For this review, take the finished solid that the model builds, in its own axes (mm). A direction names the side the tool comes from. Give positions to 0.01 mm unless a question says otherwise; leave off trailing zeros. Order: outer loops, then holes, each group sorted by start corner. A loop starts at its lowest first (then second) coordinate and runs counter-clockwise, first axis right, second up. Notation, with made-up numbers: (-8.75, 62.5) - (33.25, 62.5) arc R10 ccw to (33.25, 80.5) - close; hole circle Ø7 at (-31.5, -6). An arc over 180 degrees is marked (long way). One line per item, written item: value.
```python
from build123d import *

# Parameters (mm, degrees)
F0_R         = 25
F1_DEPTH     = 7
F2_R         = 5
F3_DEPTH     = 6
F5_DEPTH     = 8
F7_R         = 25
F7_R_2       = 24.4
F8_DEPTH     = 5
F10_DEPTH    = 25
F11_R        = 5
F12_T1_DEPTH = 7
F13_R        = 2


# Not quite as in the source:
# - a fillet or chamfer that OpenCascade refuses, or shapes differently, is made with other operations: its cross-section is extruded or revolved along the edge and cut away or added


with BuildPart() as f1:
    # F0 (on Top) → F1 (new body)
    with BuildSketch(Plane.XY):
        Circle(F0_R)
    extrude(amount=F1_DEPTH)

    # F2 (on face) → F3 (join)
    with BuildSketch(Plane.XY.offset(7)):
        Circle(F2_R)
    extrude(amount=F3_DEPTH)

    # F4 (on face) → F5 (cut)
    with BuildSketch(Plane.XY.offset(13)):
        with BuildLine():
            Line((2.005093514, 1.725), (-2.005093514, 1.725))
            ThreePointArc((-2.005093514, 1.725), (-2.645, 0), (-2.005093514, -1.725))
            Line((-2.005093514, -1.725), (2.005093514, -1.725))
            ThreePointArc((2.005093514, -1.725), (2.645, 0), (2.005093514, 1.725))
        make_face()
    extrude(amount=-F5_DEPTH, mode=Mode.SUBTRACT)

    # F7 (on offset) → F8 (cut)
    with BuildSketch(Plane.XY.offset(1)):
        Circle(F7_R)
        Circle(F7_R_2, mode=Mode.SUBTRACT)
    extrude(amount=F8_DEPTH, mode=Mode.SUBTRACT)

    # F9 (on face) → F10 (cut)
    with BuildSketch(Plane.XY.offset(7)):
        with BuildLine():
            Line((7.1352549156, 7.0062926922), (15.9346604169, 12.0866318271))
            ThreePointArc((15.9346604169, 12.0866318271), (0, 20.0000017881), (-15.9346604169, 12.0866318271))
            Line((-15.9346604169, 12.0866318271), (-7.1352549156, 7.0062926922))
            ThreePointArc((-7.1352549156, 7.0062926922), (0, 10), (7.1352549156, 7.0062926922))
        make_face()
        with BuildLine():
            ThreePointArc((2.5, -19.8431366353), (15.0000012666, -13.2287578225), (20.0000017881, 0))
            ThreePointArc((20.0000017881, 0), (19.6047610649, 3.9564397015), (18.4346604169, 7.7565048082))
            Line((18.4346604169, 7.7565048082), (9.6352549156, 2.6761656733))
            ThreePointArc((9.6352549156, 2.6761656733), (9.9083941473, 1.3504537837), (10, 0))
            ThreePointArc((10, 0), (7.9056941504, -6.123724357), (2.5, -9.6824583655))
            Line((2.5, -9.6824583655), (2.5, -19.8431366353))
        make_face()
        with BuildLine():
            ThreePointArc((-18.4346604169, 7.7565048082), (-17.3205096243, -10.0000008941), (-2.5, -19.8431366353))
            Line((-2.5, -19.8431366353), (-2.5, -9.6824583655))
            ThreePointArc((-2.5, -9.6824583655), (-8.6602540378, -5), (-9.6352549156, 2.6761656733))
            Line((-9.6352549156, 2.6761656733), (-18.4346604169, 7.7565048082))
        make_face()
    extrude(amount=-F10_DEPTH, mode=Mode.SUBTRACT)

    # F11
    f11_edges = [f1.edges().sort_by_distance(p)[0] for p in [
        (-18.43466, 7.756505, 3.5),
        (-15.93466, 12.086632, 3.5),
        (15.93466, 12.086632, 3.5),
        (18.43466, 7.756505, 3.5),
        (2.5, -19.843137, 3.5),
        (-2.5, -19.843137, 3.5),
    ]]
    fillet(f11_edges, radius=F11_R)

    # F12: fillet of radius 5 on 6 edges, made by hand

    # F12_s2 → F12_t1 (join)
    with BuildSketch(Plane.XY):
        with BuildLine():
            ThreePointArc((-12.5, 4.3301270189), (-10.6698729811, 2.5), (-10, 0))
            ThreePointArc((-10, 0), (-9.9083941473, 1.3504537837), (-9.6352549156, 2.6761656733))
            Line((-9.6352549156, 2.6761656733), (-12.5, 4.3301270189))
        make_face()
        with BuildLine():
            ThreePointArc((-2.5, -12.9903810568), (-3.1698729811, -10.4903810568), (-5, -8.6602540378))
            ThreePointArc((-5, -8.6602540378), (-3.7846697903, -9.2561479341), (-2.5, -9.6824583655))
            Line((-2.5, -9.6824583655), (-2.5, -12.9903810568))
        make_face()
        with BuildLine():
            ThreePointArc((2.5, -12.9903810568), (3.1698729811, -10.4903810568), (5, -8.6602540378))
            ThreePointArc((5, -8.6602540378), (3.7846697903, -9.2561479341), (2.5, -9.6824583655))
            Line((2.5, -9.6824583655), (2.5, -12.9903810568))
        make_face()
        with BuildLine():
            ThreePointArc((12.5, 4.3301270189), (10.6698729811, 2.5), (10, 0))
            ThreePointArc((10, 0), (9.9083941473, 1.3504537837), (9.6352549156, 2.6761656733))
            Line((9.6352549156, 2.6761656733), (12.5, 4.3301270189))
        make_face()
        with BuildLine():
            ThreePointArc((10, 8.6602540378), (7.5, 7.9903810568), (5, 8.6602540378))
            ThreePointArc((5, 8.6602540378), (6.123724357, 7.9056941504), (7.1352549156, 7.0062926922))
            Line((7.1352549156, 7.0062926922), (10, 8.6602540378))
        make_face()
        with BuildLine():
            ThreePointArc((-10, 8.6602540378), (-7.5, 7.9903810568), (-5, 8.6602540378))
            ThreePointArc((-5, 8.6602540378), (-6.123724357, 7.9056941504), (-7.1352549156, 7.0062926922))
            Line((-7.1352549156, 7.0062926922), (-10, 8.6602540378))
        make_face()
    extrude(amount=F12_T1_DEPTH)

    # F13
    f13_edges = [f1.edges().sort_by_distance(p)[0] for p in [
        (-5, 0, 7),
        (-5, 0, 13),
    ]]
    fillet(f13_edges, radius=F13_R)


solid = f1.part
```
(1) Wall thickness on line 1 (Y direction, x = -9, z = 2.75); line 2 (Y direction, x = 6, z = 1.25); line 3 (X direction, y = 9, z = 3.75): over which ranges is each line inside the solid? List them lowest first. Write a range as from..to.
Answers below:
line 1: y = -22.68..-17.76, -4.36..8.22, 17.86..22.68
line 2: y = -23.65..-17.76, -8..8.22, 19.08..23.65
line 3: x = -22.68..-10.51, -4.36..4.36, 10.51..22.68
(2) Machinability: for faces 4 (the face through (18, 4, 3)), 5 (the face through (-2.645, 0.026, 9.056)), 6 (the face through (24, -5.4, 1)), which of the approach directions +Z, -Z, +X, -X, +Y, -Y give a long, thin tool a straight path to every point of the face, cutting with its end or side? Answer none if there is none.
Answers below:
face 4: +Z, -Z
face 5: +Z
face 6: none
(3) For P1, Ø1.5, axis at x = 3, z = 11, coming from the +Y side; P2, Ø5, axis at y = -7, z = 11.5, coming from the -X side; P3, Ø4.5, axis at x = 0.5, z = 9.5, coming from the +Y side, all flat-tipped, find the tip position at first contact; note any pin that passes through.
Answers below:
P1: stops at y = 4.47
P2: stops at x = -2.12
P3: stops at y = 6.01
(4) Take a section at D-D (y = 21.5). Write out the cut boundary in (x, z).
Answers below:
outline: (-12.76, 0) - (12.76, 0) - (12.76, 1) - (11.54, 1) - (11.54, 6) - (12.76, 6) - (12.76, 7) - (-12.76, 7) - (-12.76, 6) - (-11.54, 6) - (-11.54, 1) - (-12.76, 1) - close
(5) Draft analysis for pull direction X (two halves, no side actions). For faces 1 (the face through (-1.08, -4.88, 9.99)), 2 (the face through (-7.54, 7.99, 3.45)), 3 (the face through (0, 0, 0)), state which applies: pulls with the +X half, pulls with the -X half, needs draft (parallel to the pull), parting line crosses it, or undercut.
Answers below:
face 1: parting line crosses it
face 2: undercut
face 3: needs draft
(6) Take a section at B-B (z = 9.75). Write out the cut boundary in (x, y) (3 decimals).
Answers below:
outline: circle Ø10 at (0, 0); hole (-2.005, -1.725) - (2.005, -1.725) arc R2.645 ccw to (2.005, 1.725) - (-2.005, 1.725) arc R2.645 ccw to start
(7) Take a section at A-A (x = 0). Write out the cut boundary in (y, z) (3 decimals), then the cut area to 3 significant figures.
Answers below:
outline: (-25, 0) - (10, 0) - (10, 7) - (7, 7) arc R2 cw to (5, 9) - (5, 11) arc R2 ccw to (3, 13) - (1.725, 13) - (1.725, 5) - (-1.725, 5) - (-1.725, 13) - (-3, 13) arc R2 ccw to (-5, 11) - (-5, 9) arc R2 cw to (-7, 7) - (-25, 7) - (-25, 6) - (-24.4, 6) - (-24.4, 1) - (-25, 1) - close; (20, 0) - (25, 0) - (25, 1) - (24.4, 1) - (24.4, 6) - (25, 6) - (25, 7) - (20, 7) - close
area: 306 mm^2
(8) Take a section at C-C (y = -10.5). Write out the cut boundary in (x, z).
Answers below:
outline: (-22.69, 0) - (-17.02, 0) - (-17.02, 7) - (-22.69, 7) - (-22.69, 6) - (-22.03, 6) - (-22.03, 1) - (-22.69, 1) - close; (-3.16, 0) - (3.16, 0) - (3.16, 7) - (-3.16, 7) - close; (17.02, 0) - (22.69, 0) - (22.69, 1) - (22.03, 1) - (22.03, 6) - (22.69, 6) - (22.69, 7) - (17.02, 7) - close
